Geometry check sheet. Reference: the model listing, model coordinates, mm. Coordinates: 2 decimals unless noted, no trailing zeros. Order: outer loops, then holes, each group sorted by start corner. A loop starts at its lowest first (then second) coordinate and runs counter-clockwise, first axis right, second up. Notation, with made-up numbers: M 10,12.25 L 51,12.25 A27 cw 51,48.25 Z; hole C -6.75,-39.5 d7. An arc over 180 degrees is marked long. One line per item, written item: value. Start each with the question number.
1) Go/stop test with flat-tipped pins: P1, Ø1.5, axis at x = 33.5, y = 2, coming from the -Z side; P2, Ø1.5, axis at y = 2, z = 2.5, coming from the +X side. Record where each tip stops, or that it passes through.
2) Thickness scan on L1, parallel to X at y = 0.9, z = -1; L2, parallel to X at y = 1.4, z = 0; L3, parallel to Z at x = -30, y = 1.3. Record the ranges inside material, lowest first. Write a range as from..to.
3) Sectioned sample at A-A, the plane z = 0. Enter the section's corners in (x, y).
4) Sectioned sample at B-B, the plane y = 2.5. Enter the section's corners in (x, z).
5) Sectioned sample at C-C, the plane x = -33.5. Enter the section's corners in (y, z), then the cut area to 3 significant figures.
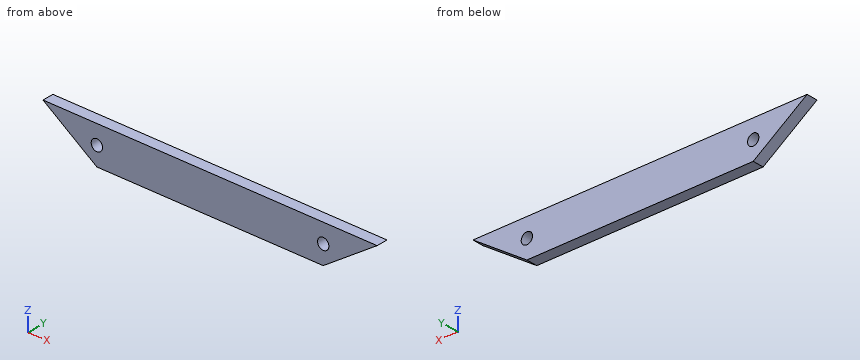
Autodesk Inventor part; units mm, degrees
ref_plane "YZ Plane" through (0, 0, 0) normal (1, 0, 0) x (0, 1, 0)
ref_plane "XZ Plane" through (0, 0, 0) normal (0, 1, 0) x (-1, 0, 0)
ref_plane "XY Plane" through (0, 0, 0) normal (0, 0, 1) x (1, 0, 0)
sketch "Эскиз1" plane through (0, 0, 0) normal (0, 1, 0) x (-1, 0, 0)
  line L0 (-30, -5) -> (30, -5)
  line L1 (30, -5) -> (30, 5)
  line L2 (30, 5) -> (-30, 5)
  line L3 (-30, 5) -> (-30, -5)
  line L4 (-30, -5) -> (30, 5) construction
  line L5 (30, -5) -> (-30, 5) construction
  line L6 (30, 5) -> (44.2815, 5)
  line L7 (30, -5) -> (44.2815, 5)
  line L8 (30, -5) -> (49.277, -5) construction
  line L9 (-30, 5) -> (-44.2815, 5)
  line L10 (-30, -5) -> (-44.2815, 5)
  line L11 (-30, -5) -> (0.6976, -5) construction
  circle A0 centre (30, 0) radius 1.5
  circle A1 centre (-30, 0) radius 1.5
  point P0 (0, 0)
  dimension "d0" = 60
  dimension "d1" = 10
  dimension "d3" = 35
  dimension "d4" = 145
  dimension "d7" = 3
  dimension "d8" = 3
extrude "Выдавливание1" add sketch "Эскиз1" along normal blind 3 contours L3 A1 L2 L1 A0 L0 | L10 L9 L3 A1 | L1 A0 L6 L7
properties part number "Flash"
Final values:
1. P1: stops at z = -3.07
1. P2: stops at x = 41.78
2. L1: x = -35.71..-31.12, -28.88..28.88, 31.12..35.71
2. L2: x = -37.14..-31.5, -28.5..28.5, 31.5..37.14
2. L3: z = -5..-1.5, 1.5..5
3. outline: M -37.14,0 L -31.5,0 L -31.5,3 L -37.14,3 Z; M -28.5,0 L 28.5,0 L 28.5,3 L -28.5,3 Z; M 31.5,0 L 37.14,0 L 37.14,3 L 31.5,3 Z
4. outline: M -44.28,5 L -30,-5 L 30,-5 L 44.28,5 Z; hole C -30,0 d3; hole C 30,0 d3
5. outline: M 0,-2.55 L 3,-2.55 L 3,5 L 0,5 Z
5. area: 22.6 mm^2
